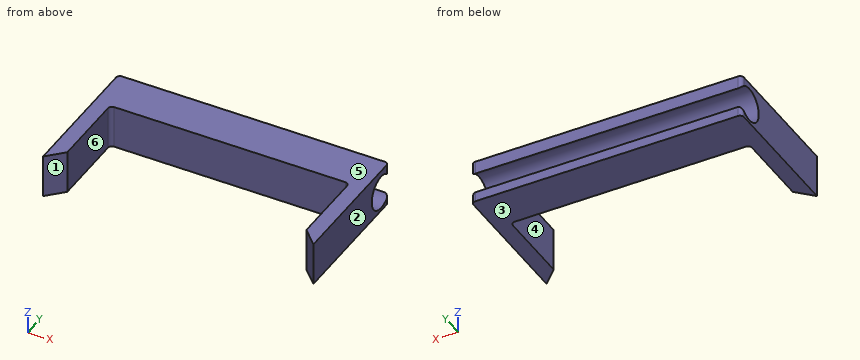
```python
from build123d import *

# Parameters (mm, degrees)
F1_DEPTH    = 11
F2_T1_DEPTH = 36.7168298797
F3_R        = 4.35
F4_DEPTH    = 69.001
F5_T1_DEPTH = 36.7168298797
F6_R        = 1


# Not quite as in the source:
# - a fillet or chamfer that OpenCascade refuses, or shapes differently, is made with other operations: its cross-section is extruded or revolved along the edge and cut away or added


with BuildPart() as f1:
    # F0 (on Top) → F1 (new body)
    with BuildSketch(Plane.XY):
        Polygon((-65, -25), (-61, -25), (-61, 0), (0, 0), (0, -25), (4, -25), (4, 11), (-65, 11), align=None)
    extrude(amount=F1_DEPTH)

    # F2: chamfer of 5 on 1 edges, made by hand

    # F2_s2 → F2_t1 (cut)
    with BuildSketch(Plane.XY.offset(-12.8584149398)):
        Polygon((0, -20), (5, -25), (0, -25), align=None)
    extrude(amount=F2_T1_DEPTH, mode=Mode.SUBTRACT)

    # F3 (on face) → F4 (cut, through all)
    with BuildSketch(Plane(origin=(-65, 0, 0), x_dir=(0, -1, 0), z_dir=(-1, 0, 0))):
        with Locations((-7.5, 5.0990604796)):
            Circle(F3_R)
    extrude(amount=-F4_DEPTH, mode=Mode.SUBTRACT)

    # F5: chamfer of 5 on 1 edges, made by hand

    # F5_s2 → F5_t1 (cut)
    with BuildSketch(Plane.XY.offset(-12.8584149398)):
        Polygon((-66, -25), (-61, -20), (-61, -25), align=None)
    extrude(amount=F5_T1_DEPTH, mode=Mode.SUBTRACT)

    # F6
    f6_edges = [f1.edges().sort_by_distance(p)[0] for p in [
        (-61, 0, 5.5),
        (0, 0, 5.5),
        (4, 11, 9.341089),
        (4, 11, 1.257971),
        (-65, 11, 9.341089),
        (-65, 11, 1.257971),
    ]]
    fillet(f6_edges, radius=F6_R)


solid = f1.part
```
For this review, take the finished solid that the model builds, in its own axes (mm). Face numbers are marked on the shaded views. A direction names the side the tool comes from. Round coordinates to 2 decimals unless told otherwise and drop trailing zeros. Loops run counter-clockwise (first coordinate to the right, second up) from the corner with the lowest first, then second, coordinate; pieces in that order, holes last.
(1) Mouldability with a two-part tool opening along X and no side actions: class the marked faces 1, 2, 3 and 4 as released by +X, released by -X, zero draft, split by the parting line, or undercut.
Returned:
face 1: undercut
face 2: released by +X
face 3: zero draft
face 4: undercut
(2) Clearance check with a flat-ended pin moving along its axis: P1, Ø5.5, axis at x = -29, z = 6.5, coming from the -Y side. State where the tip first meets the part, or that it passes through.
Returned:
P1: stops at y = 0
(3) Wall thickness on line 1 along Z through (x, y) = (-38.5, 4); line 2 along X through (y, z) = (-11, 6.25); line 3 along Z through (x, y) = (-42.5, 7.5): over which ranges is each line inside the solid? List them lowest first.
Returned:
line 1: z = 0 to 2.52, 7.68 to 11
line 2: x = -65 to -61, 0 to 4
line 3: z = 0 to 0.75, 9.45 to 11
(4) We need section C-C (y = 7.5). Give the boundary of the cut face in (x, z).
Returned:
outline: (-65, 0) - (4, 0) - (4, 0.75) - (-65, 0.75) - close; (-65, 9.45) - (4, 9.45) - (4, 11) - (-65, 11) - close
(5) We need section B-B (x = -13). Give the boundary of the cut face in (y, z).
Returned:
outline: (0, 0) - (11, 0) - (11, 2.52) arc R4.35 cw (long way) to (11, 7.68) - (11, 11) - (0, 11) - close
(6) We need section D-D (z = 5.25). Give the boundary of the cut face in (x, y).
Returned:
outline: (-65, -24) - (-61, -20) - (-61, -1) arc R1 cw to (-60, 0) - (-1, 0) arc R1 cw to (0, -1) - (0, -20) - (4, -24) - (4, 3.15) - (-65, 3.15) - close
(7) Tool access review of the marked faces 5 and 6: name each direction out of +Z, -Z, +X, -X, +Y, -Y from which nothing blocks a thin tool from reaching the whole face with its end or side.
Returned:
face 5: +Z, +X, -X, +Y, -Y
face 6: +Z, -Z, -Y
(8) We need section A-A (y = -3.5). Give the boundary of the cut face in (x, z), plus the area to 3 significant figures.
Returned:
outline: (-65, 0) - (-61, 0) - (-61, 11) - (-65, 11) - close; (0, 0) - (4, 0) - (4, 11) - (0, 11) - close
area: 88.0 mm2
